CAD build for the part. Positions are in the model's coordinates, mm. Face numbers are marked on the shaded views. Give positions to 0.01 mm unless a question says otherwise; leave off trailing zeros. Write each loop counter-clockwise with the first axis right and the second up, starting at its lowest first coordinate (ties: lowest second). Pieces come first, ordered by that corner, then holes. Notation, with made-up numbers: (71, 73) -> (103, 73) arc R16 cw to (103, 91) -> close; hole circle Ø4 at (36.5, 18). An arc over 180 degrees is marked (long way). Answer as a JSON object with one key per item and string values.
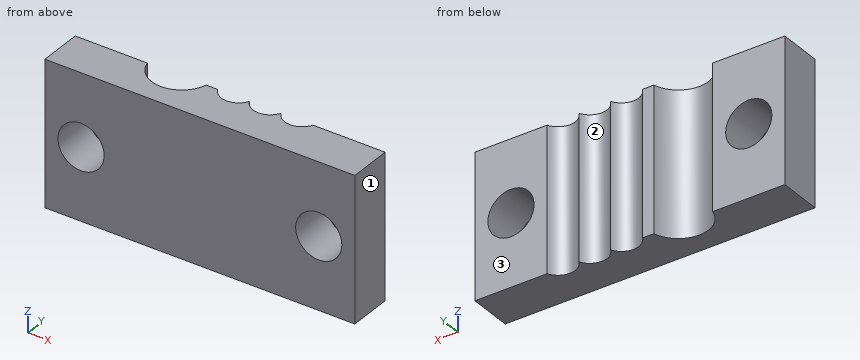
```python
from build123d import *

# Parameters (mm, degrees)
BOSS_EXTRUDE1_DEPTH = 10
SKETCH2_R           = 1.6
CUT_EXTRUDE1_DEPTH  = 24.882141932


with BuildPart() as part:
    # Sketch1 → Boss-Extrude1 (new body)
    with BuildSketch(Plane.XY):
        with BuildLine():
            Line((0, 0), (21.479215611, 0))
            Line((21.479215611, 0), (21.479215611, 3))
            Line((21.479215611, 3), (16.479215611, 3))
            ThreePointArc((16.479215611, 3), (15.379215611, 2.291695403), (14.279215611, 3))
            ThreePointArc((14.279215611, 3), (13.179215611, 2.291695403), (12.079215611, 3))
            ThreePointArc((12.079215611, 3), (10.979215611, 2.291695403), (9.879215611, 3))
            Line((9.879215611, 3), (9.079215611, 3))
            ThreePointArc((9.079215611, 3), (7.039607805, 1.4), (5, 3))
            Line((5, 3), (0, 3))
            Line((0, 3), (0, 0))
        make_face()
    extrude(amount=BOSS_EXTRUDE1_DEPTH)

    # Sketch2 → Cut-Extrude1 (cut, through all)
    with BuildSketch(Plane.XZ):
        with Locations((2.5, 5)):
            Circle(SKETCH2_R)
        with Locations((18.979215611, 5)):
            Circle(SKETCH2_R)
    extrude(amount=-CUT_EXTRUDE1_DEPTH, mode=Mode.SUBTRACT)


solid = part.part
```
1) Slice it at B-B (x = 2.5). List the corners of the cut face in (y, z), then the cut area to 3 significant figures.
Model answer:
{"outline": "(0, 0) -> (3, 0) -> (3, 3.4) -> (0, 3.4) -> close; (0, 6.6) -> (3, 6.6) -> (3, 10) -> (0, 10) -> close", "area": "20.4 mm2"}
2) Slice it at A-A (z = 5). List the corners of the cut face in (x, y).
Model answer:
{"outline": "(0, 0) -> (0.9, 0) -> (0.9, 3) -> (0, 3) -> close; (4.1, 0) -> (17.38, 0) -> (17.38, 3) -> (16.48, 3) arc R1.21 cw to (14.28, 3) arc R1.21 cw to (12.08, 3) arc R1.21 cw to (9.88, 3) -> (9.08, 3) arc R2.1 cw to (5, 3) -> (4.1, 3) -> close; (20.58, 0) -> (21.48, 0) -> (21.48, 3) -> (20.58, 3) -> close"}
3) Slice it at D-D (z = 2.5). List the corners of the cut face in (x, y).
Model answer:
{"outline": "(0, 0) -> (21.48, 0) -> (21.48, 3) -> (16.48, 3) arc R1.21 cw to (14.28, 3) arc R1.21 cw to (12.08, 3) arc R1.21 cw to (9.88, 3) -> (9.08, 3) arc R2.1 cw to (5, 3) -> (0, 3) -> close"}
4) Wall check: probe 1 along X at (y, z) = (2.8, 7); probe 2 along Z at (x, y) = (20, 0.9); probe 3 along Z at (x, y) = (2.5, 2.2). Give the ranges that are in metal, low to high.
Model answer:
{"probe 1": "x = 0 to 5.06, 9.02 to 9.99, 11.96 to 12.19, 14.16 to 14.39, 16.36 to 21.48", "probe 2": "z = 0 to 3.77, 6.23 to 10", "probe 3": "z = 0 to 3.4, 6.6 to 10"}
5) Slice it at C-C (y = 1.95). List the corners of the cut face in (x, z), then the cut area to 3 significant figures.
Model answer:
{"outline": "(0, 0) -> (5.62, 0) -> (5.62, 10) -> (0, 10) -> close; (8.46, 0) -> (21.48, 0) -> (21.48, 10) -> (8.46, 10) -> close; hole circle Ø3.2 at (2.5, 5); hole circle Ø3.2 at (18.98, 5)", "area": "170 mm2"}
6) Pin check, flat tip, straight feed: pin 1 (6 mm diameter, centred on x = 14, z = 5, fed in from -Y). Stop position of the tip, or through.
Model answer:
{"pin 1": "stops at y = 0"}
7) Mould opens along X. For the marked faces 1, 2 and 3 say: released by +X, released by -X, zero draft, split by the parting line, or undercut.
Model answer:
{"face 1": "released by +X", "face 2": "undercut", "face 3": "zero draft"}
